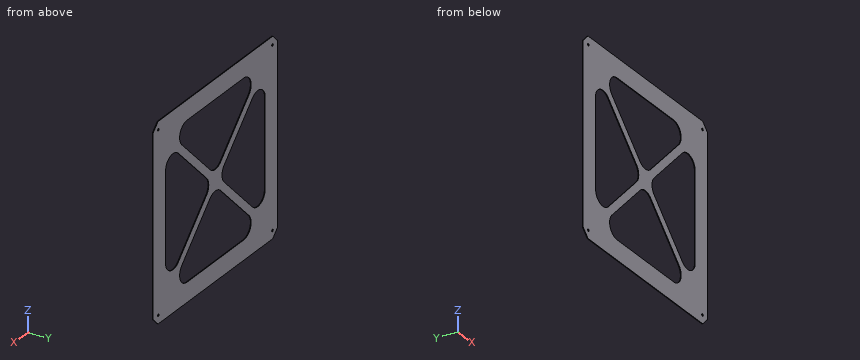
Solid Edge part; units mm, degrees
sketch "Sketch1" plane through (0, 0, 0) normal (0, -1, 0) x (1, 0, 0)
  line L0 (141.3011, -89.5112) -> (141.3011, 160.4888)
  line L1 (141.3011, 160.4888) -> (-108.6989, 160.4888)
  line L2 (-108.6989, 160.4888) -> (-108.6989, -89.5112)
  line L3 (-108.6989, -89.5112) -> (141.3011, -89.5112)
extrude "Protrusion1" add sketch "Sketch1" against normal blind 1
sketch "Sketch2" plane through (16.3011, 0, 35.4888) normal (0, -1, 0) x (1, 0, 0)
  line L0 (-10.6066, -17.6777) -> (-67.3223, -74.3934)
  arc A0 (-67.3223, -74.3934) -> (-56.7157, -100) centre (-56.7157, -85) ccw
  line L1 (56.7157, -100) -> (-56.7157, -100)
  arc A1 (67.3223, -74.3934) -> (56.7157, -100) centre (56.7157, -85) cw
  line L2 (10.6066, -17.6777) -> (67.3223, -74.3934)
  arc A2 (-10.6066, -17.6777) -> (10.6066, -17.6777) centre (0, -28.2843) cw
  line L3 (-17.6777, -10.6066) -> (-74.3934, -67.3223)
  arc A3 (-74.3934, -67.3223) -> (-100, -56.7157) centre (-85, -56.7157) cw
  line L4 (-100, -56.7157) -> (-100, 56.7157)
  arc A4 (-100, 56.7157) -> (-74.3934, 67.3223) centre (-85, 56.7157) cw
  line L5 (-74.3934, 67.3223) -> (-17.6777, 10.6066)
  arc A5 (-17.6777, 10.6066) -> (-17.6777, -10.6066) centre (-28.2843, 0) cw
  arc A6 (10.6066, 17.6777) -> (-10.6066, 17.6777) centre (0, 28.2843) cw
  line L6 (-67.3223, 74.3934) -> (-10.6066, 17.6777)
  arc A7 (-56.7157, 100) -> (-67.3223, 74.3934) centre (-56.7157, 85) ccw
  line L7 (-56.7157, 100) -> (56.7157, 100)
  arc A8 (56.7157, 100) -> (67.3223, 74.3934) centre (56.7157, 85) cw
  line L8 (67.3223, 74.3934) -> (10.6066, 17.6777)
  arc A9 (17.6777, -10.6066) -> (17.6777, 10.6066) centre (28.2843, 0) cw
  line L9 (74.3934, 67.3223) -> (17.6777, 10.6066)
  arc A10 (74.3934, 67.3223) -> (100, 56.7157) centre (85, 56.7157) cw
  line L10 (100, 56.7157) -> (100, -56.7157)
  arc A11 (74.3934, -67.3223) -> (100, -56.7157) centre (85, -56.7157) ccw
  line L11 (17.6777, -10.6066) -> (74.3934, -67.3223)
extrude "ExtrudedCutout_1" cut sketch "Sketch2" against normal blind 1
sketch "Sketch3" plane through (16.3011, 0, 35.4888) normal (0, -1, 0) x (-1, 0, 0)
  line L0 (-115, -125) -> (-125, -115)
  line L1 (-125, -125) -> (-125, -115)
  line L2 (-125, -125) -> (-115, -125)
  line L3 (-115, 125) -> (-125, 115)
  line L4 (-125, 125) -> (-125, 115)
  line L5 (-125, 125) -> (-115, 125)
  line L6 (125, 115) -> (115, 125)
  line L7 (125, 125) -> (115, 125)
  line L8 (125, 125) -> (125, 115)
  line L9 (115, -125) -> (125, -115)
  line L10 (125, -125) -> (125, -115)
  line L11 (125, -125) -> (115, -125)
extrude "ExtrudedCutout_2" cut sketch "Sketch3" against normal blind 1
sketch "Sketch4" plane through (16.3011, 1, 35.4888) normal (0, 1, 0) x (-1, 0, 0)
  circle A0 centre (114.5, -114.5) radius 1.6
  circle A1 centre (-114.5, -114.5) radius 1.6
  circle A2 centre (114.5, 114.5) radius 1.6
  circle A3 centre (-114.5, 114.5) radius 1.6
extrude "Cutout1" cut sketch "Sketch4" against normal up to next
The listing builds one solid part. Answer for the finished solid, in the listing's coordinates (mm). Coordinates: 2 decimals unless noted, no trailing zeros. Loops run counter-clockwise (first coordinate to the right, second up) from the corner with the lowest first, then second, coordinate; pieces in that order, holes last. Notation, with made-up numbers: M 46,-7.75 L 88,-7.75 A29 cw 88,20.25 Z; hole C 78,53 d4. An arc over 180 degrees is marked long. Answer in a Markdown table with one row per item.
1) Find section C-C (z = 97). Determine the outline of the cut face in (x, y).
Answers below:
| item | result |
|---|---|
| outline | M -108.7,0 L -82.91,0 L -82.91,1 L -108.7,1 Z; M -52.28,0 L -38.14,0 L -38.14,1 L -52.28,1 Z; M 70.74,0 L 84.88,0 L 84.88,1 L 70.74,1 Z; M 115.51,0 L 141.3,0 L 141.3,1 L 115.51,1 Z |
2) Find section A-A (z = 37.5). Determine the outline of the cut face in (x, y), then the cut area to 3 significant figures.
Answers below:
| item | result |
|---|---|
| outline | M -108.7,0 L -83.7,0 L -83.7,1 L -108.7,1 Z; M 2.88,0 L 29.72,0 L 29.72,1 L 2.88,1 Z; M 116.3,0 L 141.3,0 L 141.3,1 L 116.3,1 Z |
| area | 76.8 mm^2 |
3) Find section B-B (x = 12). Determine the outline of the cut face in (y, z), then the cut area to 3 significant figures.
Answers below:
| item | result |
|---|---|
| outline | M 0,-89.51 L 1,-89.51 L 1,-64.51 L 0,-64.51 Z; M 0,21.57 L 1,21.57 L 1,49.4 L 0,49.4 Z; M 0,135.49 L 1,135.49 L 1,160.49 L 0,160.49 Z |
| area | 77.8 mm^2 |
4) Find section D-D (x = -67). Determine the outline of the cut face in (y, z).
Answers below:
| item | result |
|---|---|
| outline | M 0,-89.51 L 1,-89.51 L 1,-36.13 L 0,-36.13 Z; M 0,107.11 L 1,107.11 L 1,160.49 L 0,160.49 Z |
5) Find the intervals of material crossed by probe 1 along Z at (x, y) = (131, 0.3); probe 2 along Z at (x, y) = (-14.5, 0.2); probe 3 along Z at (x, y) = (-28.5, 0.4), in increasing order.
Answers below:
| item | result |
|---|---|
| probe 1 | -89.51 to -80.6, -77.42 to 148.4, 151.58 to 160.49 |
| probe 2 | -89.51 to -64.51, -2.38 to 11.76, 59.22 to 73.36, 135.49 to 160.49 |
| probe 3 | -89.51 to -64.51, -16.38 to -2.24, 73.22 to 87.36, 135.49 to 160.49 |
